Design review of the part shown in the three views and the two pictorial views. Dimensions are in mm from the part's minimum x, y and z. A direction names the side the tool comes from. Round coordinates to 2 decimals unless told otherwise and drop trailing zeros. Order: outer loops, then holes, each group sorted by start corner. A loop starts at its lowest first (then second) coordinate and runs counter-clockwise, first axis right, second up.
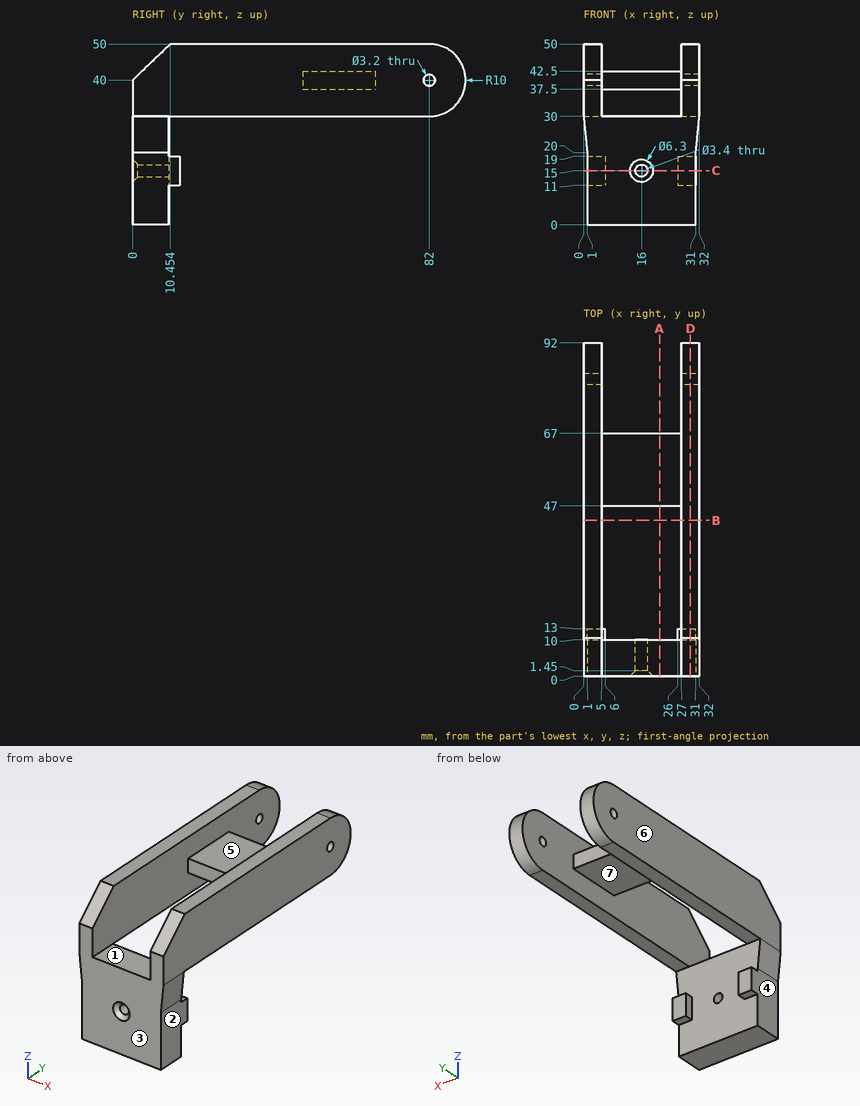
1) Take a section at B-B on y = 43. Give the boundary of the cut face in (x, z), plus the area to 3 significant figures.
Results:
outline: (0, 30) - (5, 30) - (5, 50) - (0, 50) - close; (27, 30) - (32, 30) - (32, 50) - (27, 50) - close
area: 200 mm2
2) Take a section at D-D on x = 29.5. Give the boundary of the cut face in (y, z).
Results:
outline: (0, 0) - (10, 0) - (10, 11) - (13, 11) - (13, 19) - (10, 19) - (10, 30) - (82, 30) arc R10 ccw to (82, 50) - (10.45, 50) - (0, 40) - close; hole circle Ø3.2 at (82, 40)
3) The part is to be moulded in two halves that separate along X. For the marked faces 1, 2 and 3, say which applies: released by +X, released by -X, zero draft, split by the parting line, or undercut.
Results:
face 1: undercut
face 2: released by +X
face 3: zero draft
4) For the marked faces 4, 5, 6 and 7, list the 3-axis set-ups (+Z, -Z, +X, -X, +Y, -Y) from which the entire face can be reached by the end or side of a thin tool; tool diameter is ignored.
Results:
face 4: -Z, -X, +Y, -Y
face 5: +Z, +Y, -Y
face 6: +Z, -Z, -X, +Y, -Y
face 7: -Z, +Y, -Y
5) To check wall thickness, follow line 1 along X through (y, z) = (77.5, 32.5); line 2 along Z through (x, y) = (16, 4); line 3 along Z through (x, y) = (30.1, 82). State the ranges of each line that lie inside material, in increasing order.
Results:
line 1: x = 0 to 5, 27 to 32
line 2: z = 0 to 13.3, 16.7 to 30
line 3: z = 30 to 38.4, 41.6 to 50
6) Take a section at C-C on z = 15. Give the boundary of the cut face in (x, y).
Results:
outline: (1, 0) - (12.85, 0) - (14.3, 1.45) - (14.3, 10) - (6, 10) - (6, 13) - (1, 13) - close; (17.7, 1.45) - (19.15, 0) - (31, 0) - (31, 13) - (26, 13) - (26, 10) - (17.7, 10) - close
7) Clearance check with flat-ended pins moving along their axes: P1, Ø1.5, axis at x = 16, z = 38, coming from the -Y side; P2, Ø1.5, axis at y = 12, z = 15.5, coming from the +X side; P3, Ø6.5, axis at y = 9.5, z = 6.5, coming from the -X side; P4, Ø3.5, axis at y = 82, z = 40, coming from the -X side. State where each tip first meets the part, or that it passes through.
Results:
P1: stops at y = 47
P2: stops at x = 31
P3: stops at x = 1
P4: stops at x = 0
8) Take a section at A-A on x = 21. Give the boundary of the cut face in (y, z), plus the area to 3 significant figures.
Results:
outline: (0, 0) - (10, 0) - (10, 30) - (0, 30) - close; (47, 37.5) - (67, 37.5) - (67, 42.5) - (47, 42.5) - close
area: 400 mm2
